from build123d import *

# Parameters (mm, degrees)
SKETCH1_W           = 40
SKETCH1_H           = 42
SKETCH1_R           = 12.5
BOSS_EXTRUDE1_DEPTH = 2
SKETCH3_W           = 40
SKETCH3_H           = 2
BOSS_EXTRUDE2_DEPTH = 18
BOSS_EXTRUDE3_START = -2
SKETCH4_R           = 12.5
BOSS_EXTRUDE3_DEPTH = 2
SKETCH5_R           = 12.5
CUT_EXTRUDE1_DEPTH  = 2


with BuildPart() as part:
    # Sketch1 → Boss-Extrude1 (new body)
    with BuildSketch(Plane.XY):
        Rectangle(SKETCH1_W, SKETCH1_H)
        Circle(SKETCH1_R, mode=Mode.SUBTRACT)
    extrude(amount=BOSS_EXTRUDE1_DEPTH)

    # Sketch3 → Boss-Extrude2 (add)
    with BuildSketch(Plane.XY.offset(2)):
        with Locations((0, 20)):
            Rectangle(SKETCH3_W, SKETCH3_H)
    extrude(amount=BOSS_EXTRUDE2_DEPTH)

    # Sketch4 → Boss-Extrude3 (add)
    with BuildSketch(Plane.XY.offset(2).offset(BOSS_EXTRUDE3_START)):
        Circle(SKETCH4_R)
    extrude(amount=BOSS_EXTRUDE3_DEPTH)

    # Sketch5 → Cut-Extrude1 (cut)
    with BuildSketch(Plane(origin=(0, 0, 0), x_dir=(-1, 0, 0), z_dir=(0, 0, -1))):
        Circle(SKETCH5_R)
    extrude(amount=-CUT_EXTRUDE1_DEPTH, mode=Mode.SUBTRACT)


solid = part.part
Read the model definition and answer for the solid it produces. Units are mm, in the model's axes. A direction names the side the tool comes from. Round coordinates to 2 decimals unless told otherwise and drop trailing zeros. Loops run counter-clockwise (first coordinate to the right, second up) from the corner with the lowest first, then second, coordinate; pieces in that order, holes last.
Q1. Section A-A on y = 0 is taken. Write down the section's boundary in (x, z).
Q2. Section D-D on x = -9.5 is taken. Write down the section's boundary in (y, z), and give its area (3 significant figures).
Q3. Consider probe 1 along Y at (x, z) = (3, 17.5); probe 2 along Z at (x, y) = (-3, -13.5); probe 3 along Y at (x, z) = (0, 0.9). Determine where each line is inside the solid, lowest interval first.
Q4. Each of these flat-tipped pins is pushed along its axis until it touches: pin 1 (1 mm diameter, centred on x = 14.5, y = -11, fed in from +Z); pin 2 (12 mm diameter, centred on x = 16, z = 10.5, fed in from -Y). Where does it stop, or does it pass through?
Q5. Determine the mould class of faces 1 (the face through (-20, 3, 1.8)), 2 (the face through (-11.923, 3.755, 0.986)), 3 (the face through (0, 19, 11)) for opening direction X: released by +X, released by -X, zero draft, split by the parting line, or undercut.
Q6. Which of the six approach directions +Z, -Z, +X, -X, +Y, -Y give full straight-line access (tool end or side, diameter ignored) to faces 4 (the face through (0, -21, 1)), 5 (the face through (9, -10, 2))?
Q7. Section C-C on y = 16 is taken. Write down the section's boundary in (x, z).
Q8. Section B-B on x = -0.5 is taken. Write down the section's boundary in (y, z).
Output:
1. outline: (-20, 0) - (-12.5, 0) - (-12.5, 2) - (-20, 2) - close; (12.5, 0) - (20, 0) - (20, 2) - (12.5, 2) - close
2. outline: (-21, 0) - (-8.12, 0) - (-8.12, 2) - (-21, 2) - close; (8.12, 0) - (21, 0) - (21, 20) - (19, 20) - (19, 2) - (8.12, 2) - close
2. area: 87.5 mm2
3. probe 1: y = 19 to 21
3. probe 2: z = 0 to 2
3. probe 3: y = -21 to -12.5, 12.5 to 21
4. pin 1: stops at z = 2
4. pin 2: stops at y = 19
5. face 1: released by -X
5. face 2: undercut
5. face 3: zero draft
6. face 4: +Z, -Z, +X, -X, -Y
6. face 5: +Z, +X, -X, -Y
7. outline: (-20, 0) - (20, 0) - (20, 2) - (-20, 2) - close
8. outline: (-21, 0) - (-12.49, 0) - (-12.49, 2) - (-21, 2) - close; (12.49, 0) - (21, 0) - (21, 20) - (19, 20) - (19, 2) - (12.49, 2) - close
